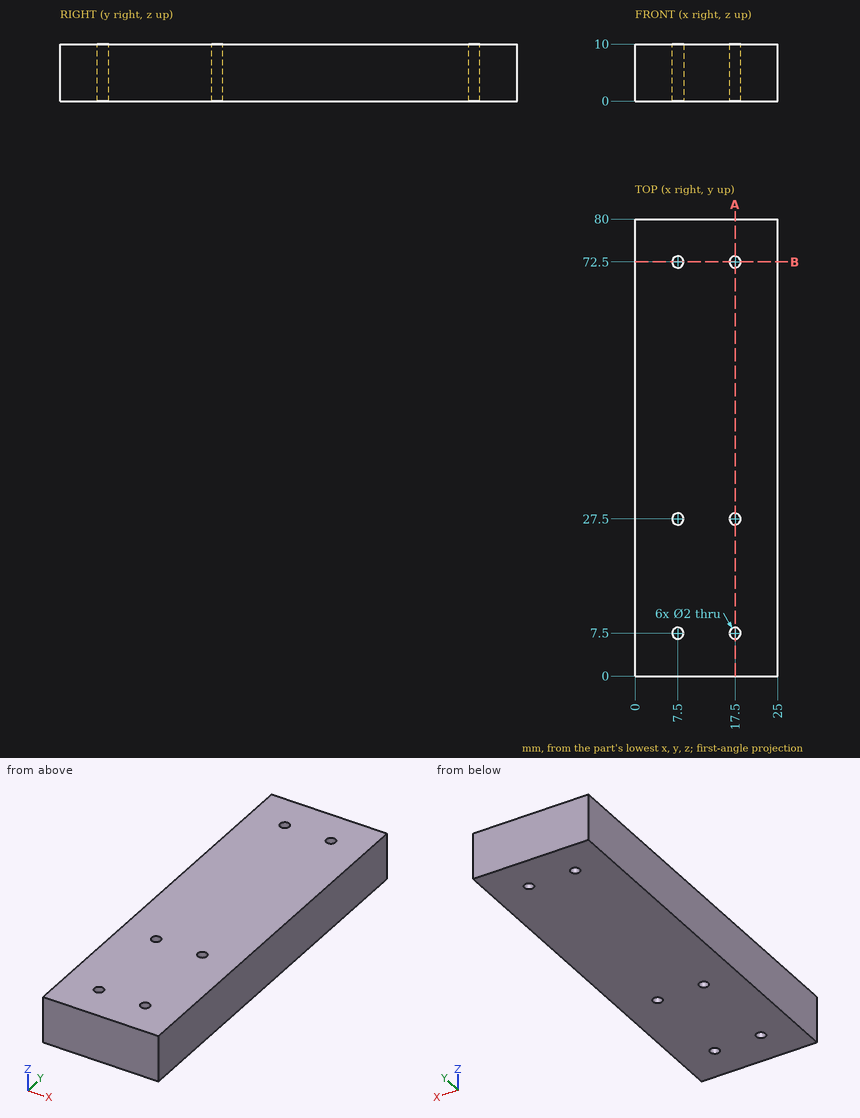
Source: three-view drawing plus pictorial views. Frame: mm from the lowest corner of the part. Coordinates: 2 decimals unless noted, no trailing zeros. Order: outer loops, then holes, each group sorted by start corner. A loop starts at its lowest first (then second) coordinate and runs counter-clockwise, first axis right, second up. Notation, with made-up numbers: M -37.5,77 L 17.5,77 A17 ccw 17.5,110 Z; hole C -34.5,30 d9. An arc over 180 degrees is marked long. Write each question's results on one line, items separated by ' | '. Start each with the question number.
1. Pin query (flat end, axial travel): pin 1 (1.2 mm diameter, centred on x = 17.5, y = 7.5, fed in from -Z). Return the tip coordinate at first contact, or that it passes through.
2. Section A-A, the plane x = 17.5. Return the cut outline in (y, z), then the cut area to 3 significant figures.
3. Section B-B, the plane y = 72.5. Return the cut outline in (x, z).
4. Material intervals for L1, parallel to Y at x = 17.5, z = 8.25; L2, parallel to X at y = 27.5, z = 3, sorted ascending.
Solution:
1) pin 1: through
2) outline: M 0,0 L 6.5,0 L 6.5,10 L 0,10 Z; M 8.5,0 L 26.5,0 L 26.5,10 L 8.5,10 Z; M 28.5,0 L 71.5,0 L 71.5,10 L 28.5,10 Z; M 73.5,0 L 80,0 L 80,10 L 73.5,10 Z | area: 740 mm²
3) outline: M 0,0 L 6.5,0 L 6.5,10 L 0,10 Z; M 8.5,0 L 16.5,0 L 16.5,10 L 8.5,10 Z; M 18.5,0 L 25,0 L 25,10 L 18.5,10 Z
4) L1: 0 to 6.5, 8.5 to 26.5, 28.5 to 71.5, 73.5 to 80 | L2: 0 to 6.5, 8.5 to 16.5, 18.5 to 25
